from build123d import *

# Parameters (mm, degrees)
SKETCH1_R                 = 14
BOSS_EXTRUDE1_DEPTH       = 20
M5X0_8_TAPPED_HOLE1_D     = 4.2
M5X0_8_TAPPED_HOLE1_DEPTH = 12.192
M5X0_8_TAPPED_HOLE1_TIP   = 1.2618073
M5X0_8_TAPPED_HOLE2_D     = 4.2
M5X0_8_TAPPED_HOLE2_DEPTH = 12.192
M5X0_8_TAPPED_HOLE2_TIP   = 1.2618073


with BuildPart() as part:
    # Sketch1 → Boss-Extrude1 (new body, symmetric)
    with BuildSketch(Plane.XY):
        Polygon((-14, 20), (-26, 8), (-26, -20), (26, -20), (26, 8), (14, 20), align=None)
        Circle(SKETCH1_R, mode=Mode.SUBTRACT)
    extrude(amount=BOSS_EXTRUDE1_DEPTH, both=True)

    # M5x0.8 Tapped Hole1
    with Locations(Plane.XY.offset(20)):
        with Locations((0, 0), (19, 0), (-19, 0), (-13.435028843, 13.435028843), (13.435028843, -13.435028843), (13.435028843, 13.435028843), (-13.435028843, -13.435028843)):
            Hole(M5X0_8_TAPPED_HOLE1_D / 2, depth=M5X0_8_TAPPED_HOLE1_DEPTH)
            with Locations((0, 0, -(M5X0_8_TAPPED_HOLE1_DEPTH + M5X0_8_TAPPED_HOLE1_TIP / 2))):  # 118° drill point
                Cone(0, M5X0_8_TAPPED_HOLE1_D / 2, M5X0_8_TAPPED_HOLE1_TIP, mode=Mode.SUBTRACT)

    # M5x0.8 Tapped Hole2
    with Locations(Plane(origin=(0, -20, 0), x_dir=(-1, 0, 0), z_dir=(0, -1, 0))):
        with Locations((20, -12), (-20, -12), (-20, 12), (20, 12)):
            Hole(M5X0_8_TAPPED_HOLE2_D / 2, depth=M5X0_8_TAPPED_HOLE2_DEPTH)
            with Locations((0, 0, -(M5X0_8_TAPPED_HOLE2_DEPTH + M5X0_8_TAPPED_HOLE2_TIP / 2))):  # 118° drill point
                Cone(0, M5X0_8_TAPPED_HOLE2_D / 2, M5X0_8_TAPPED_HOLE2_TIP, mode=Mode.SUBTRACT)


solid = part.part
Build history of the part. All positions in model axes, mm. A direction names the side the tool comes from. Coordinates: 2 decimals unless noted, no trailing zeros. Order: outer loops, then holes, each group sorted by start corner. A loop starts at its lowest first (then second) coordinate and runs counter-clockwise, first axis right, second up. Notation, with made-up numbers: M 20.5,-2 L 35.5,-2 A11 ccw 35.5,16 Z; hole C -4,51.5 d10. An arc over 180 degrees is marked long. One line per question, with ' | ' between items. Start each with the question number.
Q1. Saw through at B-B (z = -2). List the corners of the cut face in (x, y), then the cut area to 3 significant figures.
Q2. Probe L1, parallel to Y at x = 0, z = 2; L2, parallel to X at y = -10, z = -11.5; L3, parallel to X at y = -13, z = 7.5. List the from-to ranges inside material, lowest first. Write a range as from..to.
Q3. Flat gauge pins, fed straight in: pin 1 Ø4 at (x, z) = (20, -12) entering from +Y; pin 2 Ø4 at (x, y) = (-13.44, -13.44) entering from +Z; pin 3 Ø2.5 at (x, z) = (-20, 12) entering from -Y. Where does each tip first touch, or does it go through?
Q4. Saw through at C-C (y = 16.5). List the corners of the cut face in (x, z).
Q5. 3-axis set-ups, long thin cutter, end or side, ignore diameter. For faces 1 (the face through (22.003, -13.819, -12.631)), 2 (the face through (-14.56, 15.21, 13.82)), 3 (the face through (26, -6, 0)): which of +Z, -Z, +X, -X, +Y, -Y reach the whole face in a straight line?
Q6. Saw through at A-A (x = 0). List the corners of the cut face in (y, z).
Q7. Two-plate mould, pull along Z, no slides. Class faces 4 (the face through (18.636, 0.016, 6.765)), 5 (the face through (22.003, -13.819, 11.369)), 6 (the face through (-20, 14, 0)), 7 (the face through (-6, -13, -20)): +Z half, -Z half, draft (parallel to the pull), parting line (faces both ways), or undercut.
Q8. Saw through at D-D (x = -9.5). List the corners of the cut face in (y, z).
Check values:
1) outline: M -26,-20 L 26,-20 L 26,8 L 14,20 L -14,20 L -26,8 Z; hole C 0,0 d28 | area: 1,320 mm2
2) L1: y = -20..-14, 14..20 | L2: x = -26..-22.04, -17.96..-9.8, 9.8..17.96, 22.04..26 | L3: x = -26..-14.96, -11.91..-5.2, 5.2..11.91, 14.96..26
3) pin 1: stops at y = 16 | pin 2: stops at z = 7.75 | pin 3: stops at y = -7.3
4) outline: M -17.5,-20 L 17.5,-20 L 17.5,20 L -17.5,20 Z
5) face 1: -Y | face 2: +Z | face 3: +Z, -Z, +X, +Y, -Y
6) outline: M -20,-20 L -14,-20 L -14,20 L -20,20 Z; M 14,-20 L 20,-20 L 20,20 L 14,20 Z
7) face 4: +Z half | face 5: undercut | face 6: draft | face 7: -Z half
8) outline: M -20,-20 L -10.28,-20 L -10.28,20 L -20,20 Z; M 10.28,-20 L 20,-20 L 20,20 L 10.28,20 Z
